from build123d import *

# Parameters (mm, degrees)
SKETCH_1_R               = 13
EXTRUDE_1_DEPTH          = 30
SKETCH_2_R               = 13
EXTRUDE_2_DEPTH          = 45
SKETCH_3_R               = 13
SKETCH_3_R_2             = 10
CUT_EXTRUDE_1_DEPTH      = 15
SKETCH_4_R               = 9.5
CUT_EXTRUDE_2_DEPTH      = 90
CUT_EXTRUDE_3_REACH      = 97.755
CUT_EXTRUDE_3_END_RADIUS = 9.5
SKETCH_5_R               = 7.7
CUT_EXTRUDE_4_REACH      = 97.755
CUT_EXTRUDE_4_END_RADIUS = 9.5
SKETCH_6_R               = 9.5
CUT_EXTRUDE_START        = -15
SKETCH_7_R               = 13
CUT_EXTRUDE_5_DEPTH      = 15
CHAMFER_1_SIZE           = 1.2
CHAMFER_2_SIZE           = 1
CHAMFER_3_SIZE           = 0.5


with BuildPart() as part:
    # 草图1 → 拉伸1 (new, symmetric)
    with BuildSketch(Plane.XY):
        Circle(SKETCH_1_R)
    extrude(amount=EXTRUDE_1_DEPTH, both=True)

    # 草图2 → 拉伸2 (add, symmetric)
    with BuildSketch(Plane(origin=(0, 0, 0), x_dir=(0, 0, -1), z_dir=(1, 0, 0))):
        with Locations(Location((0, 0, 0), (0, 0, 270))):
            Circle(SKETCH_2_R)
    extrude(amount=EXTRUDE_2_DEPTH, both=True)

    # 草图3 → 切除-拉伸1 (cut)
    with BuildSketch(Plane(origin=(45, 0, 0), x_dir=(0, 0, -1), z_dir=(1, 0, 0))):
        with Locations(Location((0, 0, 0), (0, 0, 270))):
            Circle(SKETCH_3_R)
        Circle(SKETCH_3_R_2, mode=Mode.SUBTRACT)
    extrude(amount=-CUT_EXTRUDE_1_DEPTH, mode=Mode.SUBTRACT)

    # 草图4 → 切除-拉伸2 (cut)
    with BuildSketch(Plane.XY.offset(30)):
        Circle(SKETCH_4_R)
    extrude(amount=-CUT_EXTRUDE_2_DEPTH, mode=Mode.SUBTRACT)

    # 切除-拉伸3: up to this cylinder (the profile starts outside it)
    cut_extrude_3_end = Plane(origin=(0, 0, 0), z_dir=(0, 0, 1)) * Cylinder(CUT_EXTRUDE_3_END_RADIUS, 215.51, mode=Mode.PRIVATE)
    # 草图5 → 切除-拉伸3 (cut, up to the surface)
    with BuildSketch(Plane(origin=(45, 0, 0), x_dir=(0, 0, -1), z_dir=(1, 0, 0)), mode=Mode.PRIVATE) as cut_extrude_3_sk1:
        Circle(SKETCH_5_R)
    cut_extrude_3_tool1 = extrude(cut_extrude_3_sk1.sketch, amount=-CUT_EXTRUDE_3_REACH, mode=Mode.PRIVATE) - cut_extrude_3_end
    add(cut_extrude_3_tool1.solids().sort_by_distance((45, 0, 0))[0], mode=Mode.SUBTRACT)

    # 切除-拉伸4: up to this cylinder (the profile starts outside it)
    cut_extrude_4_end = Plane(origin=(0, 0, 0), z_dir=(0, 0, 1)) * Cylinder(CUT_EXTRUDE_4_END_RADIUS, 215.51, mode=Mode.PRIVATE)
    # 草图6 → 切除-拉伸4 (cut, up to the surface)
    with BuildSketch(Plane.ZY.offset(45), mode=Mode.PRIVATE) as cut_extrude_4_sk1:
        Circle(SKETCH_6_R)
    cut_extrude_4_tool1 = extrude(cut_extrude_4_sk1.sketch, amount=-CUT_EXTRUDE_4_REACH, mode=Mode.PRIVATE) - cut_extrude_4_end
    add(cut_extrude_4_tool1.solids().sort_by_distance((-45, 0, 0))[0], mode=Mode.SUBTRACT)

    # 草图7 → 切除-拉伸5 (cut)
    with BuildSketch(Plane.ZY.offset(45).offset(CUT_EXTRUDE_START)):
        Circle(SKETCH_7_R)
    extrude(amount=CUT_EXTRUDE_5_DEPTH, mode=Mode.SUBTRACT)

    # 倒角1
    chamfer_1_edges = [part.edges().sort_by_distance(p)[0] for p in [
        (-9.5, 0, -30),
        (-9.5, 0, 30),
        (-30, 0, -9.5),
    ]]
    chamfer(chamfer_1_edges, length=CHAMFER_1_SIZE)

    # 倒角2
    chamfer_2_edges = [part.edges().sort_by_distance(p)[0] for p in [
        (45, 0, 10),
    ]]
    chamfer(chamfer_2_edges, length=CHAMFER_2_SIZE)

    # 倒角3
    chamfer_3_edges = [part.edges().sort_by_distance(p)[0] for p in [
        (45, 0, 7.7),
    ]]
    chamfer(chamfer_3_edges, length=CHAMFER_3_SIZE)


solid = part.part
For this review, take the finished solid that the model builds, in its own axes (mm). A direction names the side the tool comes from. Round coordinates to 2 decimals unless told otherwise and drop trailing zeros. Order: outer loops, then holes, each group sorted by start corner. A loop starts at its lowest first (then second) coordinate and runs counter-clockwise, first axis right, second up. Notation, with made-up numbers: M 49,50 L 98,50 A24 cw 98,81 Z; hole C -18,-21 d11. An arc over 180 degrees is marked long. Use a Markdown table: item, result. Add a question column.
Item 1: Insertion check: pin 1 (1.5 mm diameter, centred on x = -17, y = -1, fed in from -Z); pin 2 (1.5 mm diameter, centred on y = 2, z = -22, fed in from -X); pin 3 (5 mm diameter, centred on y = -10, z = -19.5, fed in from -X). Each pin has a flat end and moves straight along its axis. Give the tip position at first contact, or say it passes through.
Item 2: Add section A-A, the plane x = -18.5. Give the boundary of the cut face in (y, z), then the cut area to 3 significant figures.
Item 3: To check wall thickness, follow line 1 along Z through (x, y) = (15.5, 0); line 2 along Y through (x, z) = (-19, 0); line 3 along Y through (x, z) = (34, 0). State the ranges of each line that lie inside material, in increasing order.
Item 4: Add section C-C, the plane y = 6.75. State how many separate pieces and enclosed holes the cut face has, then the cut area to 3 significant figures.
Item 5: Tool access review of faces 1 (the cylindrical face through (-12.987, 0.572, -18.123)), 2 (the cylindrical face through (-9.58, 8.79, 18.54)), 3 (the cylindrical face through (25.304, 7.634, 1.002)), 4 (the cylindrical face through (-18.12, 9.58, -8.79)), 5 (the cylindrical face through (37.1, -9.76, 2.17)): name each direction out of +Z, -Z, +X, -X, +Y, -Y from which nothing blocks a thin tool from reaching the whole face with its end or side.
Item 6: Mouldability with a two-part tool opening along X and no side actions: class faces 6 (the cylindrical face through (4.38, -8.43, 0.4)), 7 (the flat face through (-30, -2, -11)), 8 (the flat face through (-11, -2, -30)), 9 (the flat face through (45, -8, 3)) as released by +X, released by -X, zero draft, split by the parting line, or undercut.
Geometry results:
| question | item | result |
|---|---|---|
| 1 | pin 1 | stops at z = -13 |
| 1 | pin 2 | stops at x = -12.94 |
| 1 | pin 3 | stops at x = -10.62 |
| 2 | outline | C 0,0 d26; hole C 0,0 d19 |
| 2 | area | 247 mm² |
| 3 | line 1 | z = -13 to -7.7, 7.7 to 13 |
| 3 | line 2 | y = -13 to -9.5, 9.5 to 13 |
| 3 | line 3 | y = -10 to -7.7, 7.7 to 10 |
| 4 | separate pieces | 4 |
| 4 | enclosed holes | 0 |
| 4 | area | 988 mm² |
| 5 | face 1 | -Z |
| 5 | face 2 | +Z |
| 5 | face 3 | +X, -X |
| 5 | face 4 | -X |
| 5 | face 5 | +X |
| 6 | face 6 | undercut |
| 6 | face 7 | released by -X |
| 6 | face 8 | zero draft |
| 6 | face 9 | released by +X |
